from build123d import *

# Parameters (mm, degrees)
F1_DEPTH = 20
F3_DEPTH = 19


with BuildPart() as f1:
    # F0 (on Top) → F1 (new body)
    with BuildSketch(Plane.XY):
        Polygon((20, 10), (0, 10), (-2.12132, 7.87868), (-2.12132, -12.12132), (17.87868, -12.12132), (20, -10), align=None)
    extrude(amount=F1_DEPTH)

    # F2 (on face) → F3 (cut)
    with BuildSketch(Plane.XY.offset(20)):
        Polygon((2.787511, 7.353911), (1.65614, 6.22254), (8.93934, -1.06066), (16.22254, -8.34386), (17.353911, -7.212489), align=None)
        Polygon((8.93934, -1.06066), (1.65614, 6.22254), (0.524769, 5.091169), (15.091169, -9.475231), (16.22254, -8.34386), align=None)
    extrude(amount=-F3_DEPTH, mode=Mode.SUBTRACT)


solid = f1.part
Source: CAD feature listing. Evaluate the final solid. Frame: model axes, mm. A direction names the side the tool comes from. Give positions to 0.01 mm unless a question says otherwise; leave off trailing zeros. Write each loop counter-clockwise with the first axis right and the second up, starting at its lowest first coordinate (ties: lowest second). Pieces come first, ordered by that corner, then holes. Notation, with made-up numbers: M -30,-28 L -22,-28 A11 cw -22,-16 Z; hole C 23.25,86 d5. An arc over 180 degrees is marked long. Return JSON: item names as keys, results as strings. Group by question number.
1) Ray query, L1, parallel to Y at x = 5.25, z = 12.75; L2, parallel to Z at x = 15.25, y = -6.25; L3, parallel to Y at x = 12.25, z = 15. Return the intervals inside material, ascending.
2) Cut plane D-D, the plane x = -0.5. Output: boundary loops of the cut face in (y, z), then the cut area to 3 significant figures.
3) Cut plane C-C, the plane y = 0.75. Output: boundary loops of the cut face in (x, z), then the cut area to 3 significant figures.
4) Draft query along X for faces 3 (the face through (19, -11, 10)), 4 (the face through (7.706, -2.09, 10.633)), 5 (the face through (-2.121, -2, 10)). Return one class per face: released by +X, released by -X, zero draft, split by the parting line, or undercut.
5) Set-up query: faces 1 (the face through (9, 2, 20)), 2 (the face through (16.207, -8.36, 10.633)). Return all of +Z, -Z, +X, -X, +Y, -Y with unobstructed straight access to the full face (end or side cutting, diameter ignored); none if empty.
6) Cut plane A-A, the plane z = 11.25. Output: boundary loops of the cut face in (x, y), then the cut area to 3 significant figures.
7) Cut plane B-B, the plane x = 16.5. Output: boundary loops of the cut face in (y, z), then the cut area to 3 significant figures.
Data:
{
 "1": {"L1": "y = -12.12 to 0.37, 4.89 to 10", "L2": "z = 0 to 1", "L3": "y = -12.12 to -6.63, -2.11 to 10"},
 "2": {"outline": "M -12.12,0 L 9.5,0 L 9.5,20 L -12.12,20 Z", "area": "432 mm²"},
 "3": {"outline": "M -2.12,0 L 20,0 L 20,20 L 9.39,20 L 9.39,1 L 4.87,1 L 4.87,20 L -2.12,20 Z", "area": "356 mm²"},
 "4": {"face 3": "released by +X", "face 4": "undercut", "face 5": "released by -X"},
 "5": {"face 1": "+Z, +X, -X, +Y, -Y", "face 2": "+Z"},
 "6": {"outline": "M -2.12,-12.12 L 17.88,-12.12 L 20,-10 L 20,10 L 0,10 L -2.12,7.88 Z; hole M 0.52,5.09 L 15.09,-9.48 L 17.35,-7.21 L 2.79,7.35 Z", "area": "419 mm²"},
 "7": {"outline": "M -12.12,0 L 10,0 L 10,20 L -6.36,20 L -6.36,1 L -8.07,1 L -8.07,20 L -12.12,20 Z", "area": "410 mm²"}
}
